Read the model definition and answer for the solid it produces. Units are mm, in the model's axes. Face numbers are marked on the shaded views. A direction names the side the tool comes from. Give positions to 0.01 mm unless a question says otherwise; leave off trailing zeros. Order: outer loops, then holes, each group sorted by start corner. A loop starts at its lowest first (then second) coordinate and runs counter-clockwise, first axis right, second up. Notation, with made-up numbers: (30, -12) - (62, -12) arc R18 cw to (62, 22) - close; hole circle Ø5 at (31.25, -35). An arc over 180 degrees is marked (long way). Write item = value, one per line.
```python
from build123d import *

# Parameters (mm, degrees)
SZKIC1_R                    = 31.26
DODANIE_WYCI_GNI_CIE1_DEPTH = 30.5
SZKIC2_R                    = 19
DODANIE_WYCI_GNI_CIE2_DEPTH = 8
SZKIC3_R                    = 35.5
DODANIE_WYCI_GNI_CIE3_DEPTH = 0.5
SZKIC7_R                    = 35.5
DODANIE_WYCI_GNI_CIE4_DEPTH = 0.5
SZKIC8_R                    = 10
WYTNIJ_WYCI_GNI_CIE4_DEPTH  = 39.5


with BuildPart() as part:
    # Szkic1 → Dodanie-wyciągnięcie1 (new body)
    with BuildSketch(Plane.XY):
        Circle(SZKIC1_R)
    extrude(amount=DODANIE_WYCI_GNI_CIE1_DEPTH)

    # Szkic2 → Dodanie-wyciągnięcie2 (add)
    with BuildSketch(Plane.XY.offset(30.5)):
        Circle(SZKIC2_R)
    extrude(amount=DODANIE_WYCI_GNI_CIE2_DEPTH)

    # Szkic3 → Dodanie-wyciągnięcie3 (add)
    with BuildSketch(Plane.XY.offset(30.5)):
        Circle(SZKIC3_R)
    extrude(amount=-DODANIE_WYCI_GNI_CIE3_DEPTH)

    # Szkic7 → Dodanie-wyciągnięcie4 (add)
    with BuildSketch(Plane(origin=(0, 0, 0), x_dir=(-1, 0, 0), z_dir=(0, 0, -1))):
        Circle(SZKIC7_R)
    extrude(amount=-DODANIE_WYCI_GNI_CIE4_DEPTH)

    # Szkic8 → Wytnij-wyciągnięcie4 (cut, through all)
    with BuildSketch(Plane(origin=(0, 0, 0), x_dir=(-1, 0, 0), z_dir=(0, 0, -1))):
        Circle(SZKIC8_R)
    extrude(amount=-WYTNIJ_WYCI_GNI_CIE4_DEPTH, mode=Mode.SUBTRACT)


solid = part.part
```
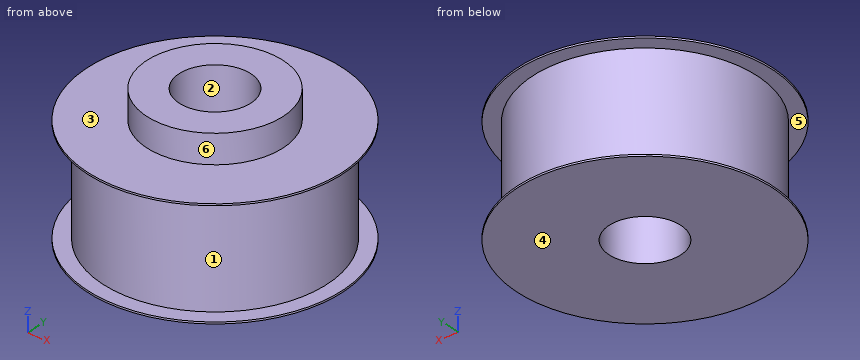
1. Flat-ended cylindrical pins translate along their axes: pin 1 (6 mm diameter, centred on x = -18.5, z = 24, fed in from -Y); pin 2 (10 mm diameter, centred on x = 16, y = 19, fed in from +Z); pin 3 (10 mm diameter, centred on x = -27.5, z = 11.5, fed in from +Y). Find the tip coordinate at first contact, or state that the pin passes through.
Recorded:
pin_1 = -27.15
pin_2 = 30.5
pin_3 = 21.7
2. Section A-A (x = 0) is taken. Determine the outline of the cut face in (y, z).
Recorded:
outline = (-35.5, 0) - (-10, 0) - (-10, 38.5) - (-19, 38.5) - (-19, 30.5) - (-35.5, 30.5) - (-35.5, 30) - (-31.26, 30) - (-31.26, 0.5) - (-35.5, 0.5) - close; (10, 0) - (35.5, 0) - (35.5, 0.5) - (31.26, 0.5) - (31.26, 30) - (35.5, 30) - (35.5, 30.5) - (19, 30.5) - (19, 38.5) - (10, 38.5) - close
3. Section C-C (z = 6) is taken. Determine the outline of the cut face in (x, y).
Recorded:
outline = circle Ø62.52 at (0, 0); hole circle Ø20 at (0, 0)
4. Section D-D (y = 27.5) is taken. Determine the outline of the cut face in (x, z).
Recorded:
outline = (-22.45, 0) - (22.45, 0) - (22.45, 0.5) - (14.86, 0.5) - (14.86, 30) - (22.45, 30) - (22.45, 30.5) - (-22.45, 30.5) - (-22.45, 30) - (-14.86, 30) - (-14.86, 0.5) - (-22.45, 0.5) - close
5. For the marked faces 4, 5 and 6, determine the directions among +Z, -Z, +X, -X, +Y, -Y from which every point of the face is accessible in a straight line to the end or side of a thin tool.
Recorded:
face_4 = -Z, +X, -X, +Y, -Y
face_5 = none
face_6 = +Z
6. Straight lines are drawn through the part: L1, parallel to Z at x = 28, y = -20; L2, parallel to Y at x = 0, z = 11; L3, parallel to Z at x = 13, y = 28. For each, find the intervals that lie inside material, in ascending order. Write a range as [from, to].
Recorded:
L1 = [0, 0.5], [30, 30.5]
L2 = [-31.26, -10], [10, 31.26]
L3 = [0, 30.5]
7. Determine the mould class of the marked faces 1, 2 and 3 for opening direction Y: +Y half, -Y half, draft (parallel to the pull), parting line (faces both ways), or undercut.
Recorded:
face_1 = parting line
face_2 = undercut
face_3 = draft
